CAD build for the part. Positions are in the model's coordinates, mm. A direction names the side the tool comes from. Coordinates: 2 decimals unless noted, no trailing zeros. Order: outer loops, then holes, each group sorted by start corner. A loop starts at its lowest first (then second) coordinate and runs counter-clockwise, first axis right, second up. Notation, with made-up numbers: (65.5, 39) -> (122.5, 39) arc R26 ccw to (122.5, 54) -> close; hole circle Ø1 at (40, 85). An arc over 180 degrees is marked (long way). Use one line per item in the form item = value. Start each with the question number.
from build123d import *

# Parameters (mm, degrees)
SKETCH2_W           = 4.7625
SKETCH2_H           = 6.95
SKETCH2_W_2         = 1.5875
SKETCH2_H_2         = 3.845
SKETCH2_W_3         = 17.78
SKETCH3_R           = 11.338051479
CUT_EXTRUDE1_DEPTH  = 21.336
SKETCH5_R           = 2
CUT_EXTRUDE3_DEPTH  = 27.432
BOSS_EXTRUDE2_START = -4.7625
SKETCH5_3_R         = 2
BOSS_EXTRUDE2_DEPTH = 4.7625
FILLET1_R           = 0.79375
CUT_EXTRUDE4_START  = -14.224
CUT_EXTRUDE4_DEPTH  = 14.224
FILLET2_R           = 0.79375


with BuildPart() as part:
    # Sketch2 → Revolve2 (revolve)
    with BuildSketch(Plane(origin=(0, 0, 0), x_dir=(0, 1, 0), z_dir=(0, 0, 1)), mode=Mode.PRIVATE) as revolve2_sk:
        with Locations((-12.85875, 3.475)):
            Rectangle(SKETCH2_W, SKETCH2_H)
        with Locations((-9.68375, 3.475)):
            Rectangle(SKETCH2_W_2, SKETCH2_H)
        with Locations((-9.68375, 8.8725)):
            Rectangle(SKETCH2_W_2, SKETCH2_H_2)
        with Locations((0, 3.475)):
            Rectangle(SKETCH2_W_3, SKETCH2_H)
        with Locations((9.68375, 3.475)):
            Rectangle(SKETCH2_W_2, SKETCH2_H)
        with Locations((9.68375, 8.8725)):
            Rectangle(SKETCH2_W_2, SKETCH2_H_2)
        with Locations((12.85875, 3.475)):
            Rectangle(SKETCH2_W, SKETCH2_H)
    revolve(revolve2_sk.sketch.rotate(Axis((0, -15.24, 0), (0, 1, 0)), 180), axis=Axis((0, -15.24, 0), (0, 1, 0)))

    # Sketch3 → Cut-Extrude1 (cut)
    with BuildSketch(Plane(origin=(0, 0, 0), x_dir=(-1, 0, 0), z_dir=(0, 1, 0))):
        Circle(SKETCH3_R)
    extrude(amount=-CUT_EXTRUDE1_DEPTH, mode=Mode.SUBTRACT)

    # Sketch5 → Cut-Extrude3 (cut)
    with BuildSketch(Plane(origin=(0, 15.24, 0), x_dir=(-1, 0, 0), z_dir=(0, 1, 0))):
        with Locations((-3.175, 0)):
            Circle(SKETCH5_R)
        with BuildLine():
            ThreePointArc((-1.175, 0), (-1.559736192, 1.179373914), (-2.565922829, 1.905))
            Line((-2.565922829, 1.905), (-3.784077171, 1.905))
            ThreePointArc((-3.784077171, 1.905), (-4.354373914, -1.615263808), (-1.175, 0))
        make_face()
        with BuildLine():
            Line((-3.784077171, 1.905), (-2.565922829, 1.905))
            ThreePointArc((-2.565922829, 1.905), (-3.175, 2), (-3.784077171, 1.905))
        make_face()
    extrude(amount=-CUT_EXTRUDE3_DEPTH, mode=Mode.SUBTRACT)

    # Sketch5<3> → Boss-Extrude2 (add)
    with BuildSketch(Plane(origin=(0, 15.24, 0), x_dir=(-1, 0, 0), z_dir=(0, 1, 0)).offset(BOSS_EXTRUDE2_START)):
        with BuildLine():
            Line((-15.875, -10.795), (0, -10.795))
            Line((0, -10.795), (0, -6.95))
            ThreePointArc((0, -6.95), (-5.547172703, -4.187048483), (-6.683821886, 1.905))
            Line((-6.683821886, 1.905), (-15.875, 1.905))
            Line((-15.875, 1.905), (-15.875, -10.795))
        make_face()
        with Locations((-8.255, -5.08)):
            Circle(SKETCH5_3_R, mode=Mode.SUBTRACT)
    extrude(amount=BOSS_EXTRUDE2_DEPTH)

    # Fillet1
    # the kernel refuses this fillet: 0.79375 mm, written as the material it adds along each edge
    with BuildSketch(Plane(origin=(0, 10.4775, -6.95), x_dir=(-0.9986823309895368, 0, 0.051318629846335534), z_dir=(0, 1, 0))) as fillet1_piece_1:
        with BuildLine():
            CenterArc((0.754063117, -0.7927041), FILLET1_R, 92.941633047, 84.116733906)
            Line((-0.038640983, -0.751969938), (0, 0))
            ThreePointArc((0, 0), (0.356664477, -0.0091578), (0.713328955, 0))
        make_face()
    extrude(amount=4.7625)
    with BuildSketch(Plane(origin=(6.683821886, 9.041391923, 1.905), x_dir=(1, 0, 0), z_dir=(0, 1, 0))) as fillet1_piece_2:
        with BuildLine():
            CenterArc((0.574443231, -0.79375), FILLET1_R, 90, 69.603984808)
            ThreePointArc((-0.169543589, -0.51712268), (-0.079708314, -0.26022145), (0, 0))
            Line((0, 0), (0.574443231, 0))
        make_face()
    extrude(amount=6.198608077)
    # the kernel refuses this fillet: 0.79375 mm, written as the material it takes off along each edge
    with BuildSketch(Plane(origin=(0, 10.4775, -10.795), x_dir=(1, 0, 0), z_dir=(0, 1, 0))) as fillet1_2_piece_1:
        with BuildLine():
            CenterArc((FILLET1_R, -FILLET1_R), FILLET1_R, 90, 90)
            Line((0, -FILLET1_R), (0, 0))
            Line((0, 0), (FILLET1_R, 0))
        make_face()
    extrude(amount=6.746875, mode=Mode.SUBTRACT)
    with BuildSketch(Plane(origin=(15.875, 8.493125, 1.905), x_dir=(0, 0, -1), z_dir=(0, 1, 0)), Plane(origin=(15.875, 8.493125, -10.795), x_dir=(-1, 0, 0), z_dir=(0, 1, 0))) as fillet1_2_piece_2:
        with BuildLine():
            CenterArc((FILLET1_R, FILLET1_R), FILLET1_R, 180, 90)
            Line((0, FILLET1_R), (0, 0))
            Line((0, 0), (FILLET1_R, 0))
        make_face()
    extrude(amount=8.73125, mode=Mode.SUBTRACT)

    # Sketch6 → Cut-Extrude4 (cut)
    with BuildSketch(Plane(origin=(0, 10.4775, 0), x_dir=(-1, 0, 0), z_dir=(0, 1, 0)).offset(CUT_EXTRUDE4_START)):
        with BuildLine():
            ThreePointArc((-6.514278297, 2.42212268), (-3.966657748, 5.70684907), (0, 6.95))
            Line((0, 6.95), (0, 10.795))
            ThreePointArc((0, 10.795), (-6.927032193, 8.279387055), (-10.625582337, 1.905))
            Line((-10.625582337, 1.905), (-7.258265116, 1.905))
            ThreePointArc((-7.258265116, 1.905), (-6.805238557, 2.046978568), (-6.514278297, 2.42212268))
        make_face()
    extrude(amount=CUT_EXTRUDE4_DEPTH, mode=Mode.SUBTRACT)

    # Fillet2
    # the kernel refuses this fillet: 0.79375 mm, written as the material it adds along each edge
    with BuildSketch(Plane(origin=(0, 8.89, 6.95), x_dir=(0.9986823309895368, 0, -0.051318629846333855), z_dir=(0, 1, 0))) as fillet2_piece_1:
        with BuildLine():
            CenterArc((0.754063117, -0.7927041), FILLET2_R, 92.941633047, 84.116733906)
            Line((-0.038640983, -0.751969938), (0, 0))
            ThreePointArc((0, 0), (0.356664477, -0.0091578), (0.713328955, 0))
        make_face()
    extrude(amount=1.5875)
    # the kernel refuses this fillet: 0.79375 mm, written as the material it takes off along each edge
    with BuildSketch(Plane(origin=(0, 6.746443854, 10.795), x_dir=(0, 0, -1), z_dir=(0, 1, 0))) as fillet2_2_piece_1:
        with BuildLine():
            CenterArc((0.825297773, 0.79375), FILLET2_R, 175.447928579, 94.552071421)
            ThreePointArc((0.034051564, 0.856746032), (0.00851625, 0.428711229), (0, 0))
            Line((0, 0), (0.825297773, 0))
        make_face()
    extrude(amount=5.874612291, mode=Mode.SUBTRACT)
    with BuildSketch(Plane(origin=(10.625582337, 7.107567927, 1.905), x_dir=(-1, 0, 0), z_dir=(0, 1, 0))) as fillet2_2_piece_2:
        with BuildLine():
            CenterArc((0.686260177, -0.79375), FILLET2_R, 90, 83.620629792)
            ThreePointArc((-0.102574915, -0.705555556), (-0.057113988, -0.351930706), (0, 0))
            Line((0, 0), (0.686260177, 0))
        make_face()
    extrude(amount=3.369932073, mode=Mode.SUBTRACT)


with BuildPart() as body_2:
    # Mirror1: mirrored copy
    add(part.part.mirror(Plane.ZX))


solid = body_2.part
1) Cut at D-D on z = -2.5. Give the cut face in (x, y) (1 decimal).
2) Two-plate mould, pull along Z, no slides. Class faces 5 (the face through (8, -13, -10.795)), 6 (the face through (9.84, -12.83, -6.3)), 7 (the face through (0, 0, 0)): released by +Z, released by -Z, zero draft, split by the parting line, or undercut.
3) Cut at B-B on y = -13. Count the separate pieces of the cut face and the enclosed holes in it, then the cut area to 3 significant figures.
4) Drop flat-ended pins along their axis: P1, Ø1.1, axis at x = 8.5, z = -4.5, coming from the -Y side; P2, Ø5, axis at x = 9.5, y = -12, coming from the +Z side; P3, Ø3.5, axis at x = 3.175, z = 0, coming from the +Y side; P4, Ø0.8, axis at y = -9.5, z = 8.5, coming from the +X side. Give the stop position or say it passes through.
5) Probe L1, parallel to Y at x = -9, z = 3.5; L2, parallel to Y at x = 13.5, z = 1; L3, parallel to X at y = -12.5, z = -1.75 (3 decimals). List the from-to ranges inside material, lowest first.
6) Cut at C-C on y = -5.75. Give the cut face in (x, z) (3 decimals).
7) 3-axis set-ups, long thin cutter, end or side, ignore diameter. For faces 1 (the face through (0, -13, -9)), 2 (the face through (-7, -8.89, -2)), 3 (the face through (11, -13, 1.905)), 4 (the face through (8, -10.478, -5)): which of +Z, -Z, +X, -X, +Y, -Y reach the whole face in a straight line?
Values follow:
q1.outline = (-10.5, -10.5) -> (-6.5, -10.5) -> (-6.5, -15.2) -> (15.9, -15.2) -> (15.9, -10.5) -> (10.5, -10.5) -> (10.5, -8.9) -> (6.5, -8.9) -> (6.5, 0) -> (-6.5, 0) -> (-6.5, -8.9) -> (-10.5, -8.9) -> close
q2.face_5 = released by -Z
q2.face_6 = undercut
q2.face_7 = zero draft
q3.separate_pieces = 1
q3.enclosed_holes = 2
q3.area = 277 mm^2
q4.P1 = -10.48
q4.P2 = 1.95
q4.P3 = through
q4.P4 = 0
q5.L1 = -10.48 to -8.89
q5.L2 = -15.24 to -10.48
q5.L3 = -6.726 to 2.207, 4.143 to 15.875
q6.outline = circle Ø13.9 at (0, 0); hole circle Ø4 at (3.175, 0)
q7.face_1 = -Z, -X, -Y
q7.face_2 = +Y
q7.face_3 = +Z, +X, +Y, -Y
q7.face_4 = -Y
